Input: dimensioned drawing with shaded views. Units: mm. Origin: part minimum x, y, z. A direction names the side the tool comes from. Give positions to 0.01 mm unless a question says otherwise; leave off trailing zeros. Order: outer loops, then holes, each group sorted by start corner. A loop starts at its lowest first (then second) coordinate and runs counter-clockwise, first axis right, second up. Notation, with made-up numbers: (53.5, 69) -> (93.5, 69) arc R35 cw to (93.5, 102) -> close; hole circle Ø4 at (10, -34). An arc over 180 degrees is marked (long way). One line per question, with ' | ' between items. Start each with the question number.
(1) First-contact query: pin 1 Ø3 at (y, z) = (11.5, 10.5) entering from +X; pin 2 Ø12 at (y, z) = (16, 16) entering from +X; pin 3 Ø11 at (y, z) = (11.5, 13) entering from -X; pin 4 Ø3 at (y, z) = (26.5, 22.5) entering from +X. Flat tips, straight axial feed; report the tip coordinate or a pass-through.
(2) Section C-C (x = 12.7). Return loops of the section in (y, z), then the cut area to 3 significant figures.
(3) Section B-B (z = 12.7). Return loops of the section in (x, y), then the cut area to 3 significant figures.
(4) Set-up query: the marked faces 1, 2, 3 and 4. Return all of +Z, -Z, +X, -X, +Y, -Y with unobstructed straight access to the full face (end or side cutting, diameter ignored); none if empty.
(5) Section D-D (y = 29). Return loops of the section in (x, z), then the cut area to 3 significant figures.
(6) Ray query, L1, parallel to Y at x = 14, z = 12.7; L2, parallel to Z at x = 12.75, y = 12.7; L3, parallel to X at y = 22, z = 11. Return the intervals inside material, ascending.
(7) Section A-A (y = 12.7). Return loops of the section in (x, z).
(8) Mould query, pull axis Z, two halves, no side actions, for the marked faces 5, 6 and 7. Classes: +Z half, -Z half, draft (parallel to the pull), parting line (faces both ways), or undercut.
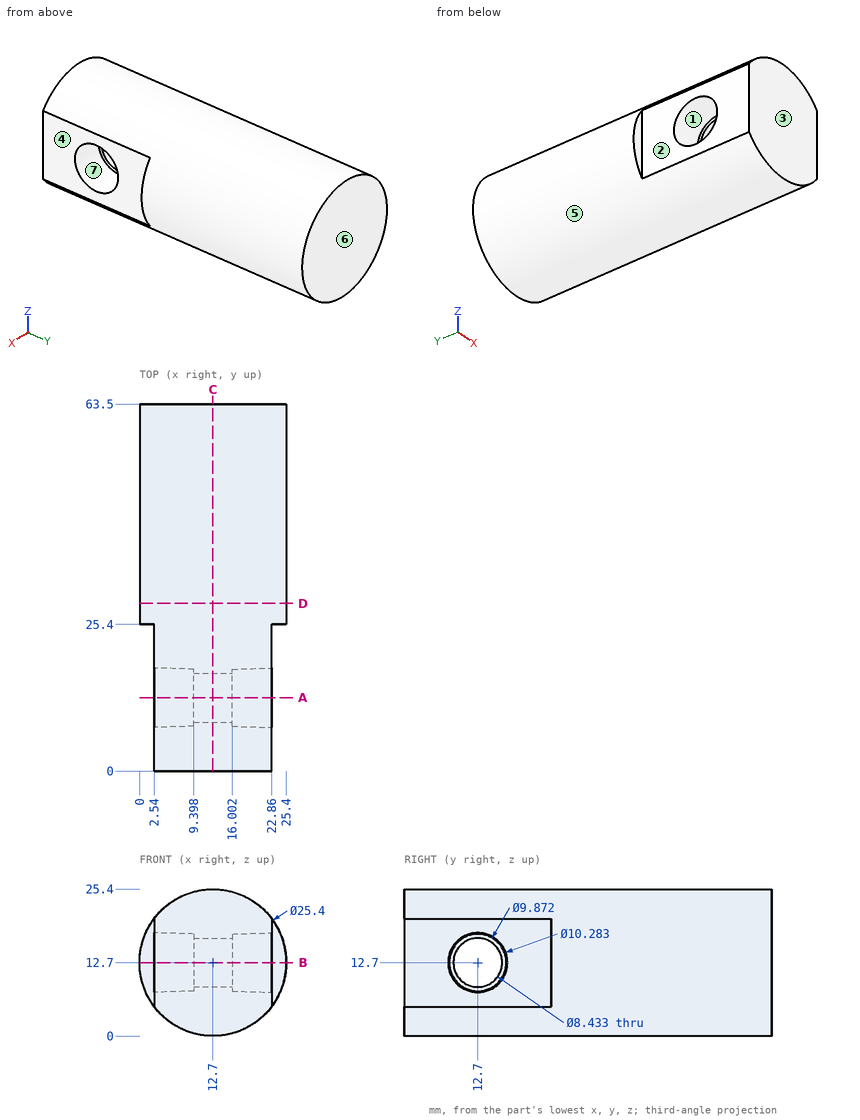
Response:
1) pin 1: passes through | pin 2: stops at x = 22.86 | pin 3: stops at x = 2.54 | pin 4: stops at x = 22.31
2) outline: (0, 0) -> (63.5, 0) -> (63.5, 25.4) -> (0, 25.4) -> close; hole circle Ø8.43 at (12.7, 12.7) | area: 1,560 mm^2
3) outline: (0, 25.4) -> (2.54, 25.4) -> (2.54, 17.84) -> (9.4, 17.64) -> (9.4, 16.92) -> (16, 16.92) -> (16, 17.64) -> (22.86, 17.84) -> (22.86, 25.4) -> (25.4, 25.4) -> (25.4, 63.5) -> (0, 63.5) -> close; (2.54, 0) -> (22.86, 0) -> (22.86, 7.56) -> (16, 7.76) -> (16, 8.48) -> (9.4, 8.48) -> (9.4, 7.76) -> (2.54, 7.56) -> close | area: 1,290 mm^2
4) face 1: -X | face 2: +Z, -Z, -X, -Y | face 3: +Z, -Z, +X, -X, -Y | face 4: +Z, -Z, +X, -Y
5) outline: circle Ø25.4 at (12.7, 12.7) | area: 507 mm^2
6) L1: y = 0 to 8.48, 16.92 to 63.5 | L2: z = 0 to 8.48, 16.92 to 25.4 | L3: x = 2.54 to 22.86
7) outline: (2.54, 5.08) arc R12.7 ccw to (22.86, 5.08) -> (22.86, 7.56) -> (16, 7.76) -> (16, 8.48) -> (9.4, 8.48) -> (9.4, 7.76) -> (2.54, 7.56) -> close; (2.54, 17.84) -> (9.4, 17.64) -> (9.4, 16.92) -> (16, 16.92) -> (16, 17.64) -> (22.86, 17.84) -> (22.86, 20.32) arc R12.7 ccw to (2.54, 20.32) -> close
8) face 5: parting line | face 6: draft | face 7: undercut
